```python
from build123d import *

# Parameters (mm, degrees)
SKETCH007_R      = 2.25
EXTRUDE007_DEPTH = 6
SKETCH006_R      = 3
SKETCH006_W      = 15
SKETCH006_H      = 10
EXTRUDE006_DEPTH = 2
SKETCH005_W      = 62
SKETCH005_H      = 5
EXTRUDE005_DEPTH = 2
SKETCH004_W      = 62
SKETCH004_H      = 5
EXTRUDE004_DEPTH = 2
SKETCH003_R      = 1
EXTRUDE003_DEPTH = 4
SKETCH002_R      = 3
EXTRUDE002_DEPTH = 4
SKETCH001_W      = 88
SKETCH001_H      = 84
EXTRUDE001_DEPTH = 29
SKETCH_W         = 91
SKETCH_H         = 87
EXTRUDE_DEPTH    = 29
BOX_W            = 91
BOX_H            = 87
BOX_DEPTH        = 3
FILLET_R         = 2
FILLET001_R      = 2
FILLET002_R      = 2
FILLET003_R      = 2
FILLET004_R      = 2
FILLET005_R      = 2
FILLET006_R      = 2
FILLET007_R      = 2
FILLET008_R      = 2
FILLET009_R      = 2
FILLET010_R      = 2
FILLET011_R      = 2


with BuildPart() as extrude007:
    # Sketch007 (on Face52 of Fillet011) → Extrude007 (new body)
    with BuildSketch(Plane(origin=(0, 0, 0), x_dir=(1, 0, 0), z_dir=(0, 0, -1))):
        with Locations((45.5, -5.25)):
            Circle(SKETCH007_R)
        with Locations((75.5, -5.25)):
            Circle(SKETCH007_R)
        with Locations((15.5, -5.25)):
            Circle(SKETCH007_R)
        with Locations((15.5, -35.25)):
            Circle(SKETCH007_R)
        with Locations((45.5, -35.25)):
            Circle(SKETCH007_R)
        with Locations((75.5, -35.25)):
            Circle(SKETCH007_R)
        with Locations((15.5, -65.25)):
            Circle(SKETCH007_R)
        with Locations((45.5, -65.25)):
            Circle(SKETCH007_R)
        with Locations((75.5, -65.25)):
            Circle(SKETCH007_R)
    extrude(amount=EXTRUDE007_DEPTH)


with BuildPart() as extrude006:
    # Sketch006 (on Face13 of Cut002) → Extrude006 (new body)
    with BuildSketch(Plane(origin=(0, 87, 0), x_dir=(-1, 0, 0), z_dir=(0, 1, 0))):
        with Locations((-64.5, 19.802082)):
            Circle(SKETCH006_R)
        with Locations((-45.5, 22)):
            Rectangle(SKETCH006_W, SKETCH006_H)
    extrude(amount=-EXTRUDE006_DEPTH)


with BuildPart() as extrude005:
    # Sketch005 (on Face17 of Cut001) → Extrude005 (new body)
    with BuildSketch(Plane(origin=(0, 0, 0), x_dir=(0, -1, 0), z_dir=(-1, 0, 0))):
        with Locations((-39, 10.5)):
            Rectangle(SKETCH005_W, SKETCH005_H)
    extrude(amount=-EXTRUDE005_DEPTH)


with BuildPart() as extrude004:
    # Sketch004 (on Face10 of Fusion002) → Extrude004 (new body)
    with BuildSketch(Plane.YZ.offset(91)):
        with Locations((39, 10.5)):
            Rectangle(SKETCH004_W, SKETCH004_H)
    extrude(amount=-EXTRUDE004_DEPTH)


with BuildPart() as extrude003:
    # Sketch003 (on Face34 of Fusion001) → Extrude003 (new body)
    with BuildSketch(Plane.XY.offset(7)):
        with Locations((5.302703, 5.215435)):
            Circle(SKETCH003_R)
        with Locations((85.638989, 5.056605)):
            Circle(SKETCH003_R)
        with Locations((85.765417, 81.797994)):
            Circle(SKETCH003_R)
        with Locations((5.093359, 81.86968)):
            Circle(SKETCH003_R)
    extrude(amount=EXTRUDE003_DEPTH)


with BuildPart() as extrude002:
    # Sketch002 (on Face18 of Fillet007) → Extrude002 (new body)
    with BuildSketch(Plane.XY.offset(3)):
        with Locations((5.093359, 81.86968)):
            Circle(SKETCH002_R)
        with Locations((85.80056, 81.783242)):
            Circle(SKETCH002_R)
        with Locations((5.279273, 5.214621)):
            Circle(SKETCH002_R)
        with Locations((85.631504, 5.092482)):
            Circle(SKETCH002_R)
    extrude(amount=EXTRUDE002_DEPTH)


with BuildPart() as extrude001:
    # Sketch001 (on Face6 of Box) → Extrude001 (new body)
    with BuildSketch(Plane.XY.offset(3)):
        with Locations((45.5, 43.5)):
            Rectangle(SKETCH001_W, SKETCH001_H)
    extrude(amount=EXTRUDE001_DEPTH)


with BuildPart() as cut:
    # Sketch (on Face6 of Box) → Extrude (new body)
    with BuildSketch(Plane.XY.offset(3)):
        with Locations((45.5, 43.5)):
            Rectangle(SKETCH_W, SKETCH_H)
    extrude(amount=EXTRUDE_DEPTH)

    # Cut: cut Extrude001
    add(extrude001.part, mode=Mode.SUBTRACT)


with BuildPart() as esp_case_bottom:
    # Box → Box (new body)
    with BuildSketch(Plane.XY):
        with Locations((45.5, 43.5)):
            Rectangle(BOX_W, BOX_H)
    extrude(amount=BOX_DEPTH)

    # Fusion: union Cut
    add(cut.part)

    # Fillet
    fillet_edges = [esp_case_bottom.edges().sort_by_distance(p)[0] for p in [
        (0, 87, 1.5),
        (0, 87, 17.5),
    ]]
    fillet(fillet_edges, radius=FILLET_R)

    # Fillet001
    fillet001_edges = [esp_case_bottom.edges().sort_by_distance(p)[0] for p in [
        (1.5, 85.5, 17.5),
    ]]
    fillet(fillet001_edges, radius=FILLET001_R)

    # Fillet002
    fillet002_edges = [esp_case_bottom.edges().sort_by_distance(p)[0] for p in [
        (0, 0, 17.5),
    ]]
    fillet(fillet002_edges, radius=FILLET002_R)

    # Fillet003
    fillet003_edges = [esp_case_bottom.edges().sort_by_distance(p)[0] for p in [
        (91, 0, 17.5),
    ]]
    fillet(fillet003_edges, radius=FILLET003_R)

    # Fillet004
    fillet004_edges = [esp_case_bottom.edges().sort_by_distance(p)[0] for p in [
        (91, 87, 17.5),
    ]]
    fillet(fillet004_edges, radius=FILLET004_R)

    # Fillet005
    fillet005_edges = [esp_case_bottom.edges().sort_by_distance(p)[0] for p in [
        (89.5, 85.5, 17.5),
    ]]
    fillet(fillet005_edges, radius=FILLET005_R)

    # Fillet006
    fillet006_edges = [esp_case_bottom.edges().sort_by_distance(p)[0] for p in [
        (89.5, 1.5, 17.5),
    ]]
    fillet(fillet006_edges, radius=FILLET006_R)

    # Fillet007
    fillet007_edges = [esp_case_bottom.edges().sort_by_distance(p)[0] for p in [
        (1.5, 1.5, 17.5),
    ]]
    fillet(fillet007_edges, radius=FILLET007_R)

    # Fusion001: union Extrude002
    add(extrude002.part)

    # Fusion002: union Extrude003
    add(extrude003.part)

    # Cut001: cut Extrude004
    add(extrude004.part, mode=Mode.SUBTRACT)

    # Cut002: cut Extrude005
    add(extrude005.part, mode=Mode.SUBTRACT)

    # Cut003: cut Extrude006
    add(extrude006.part, mode=Mode.SUBTRACT)

    # Fillet008
    fillet008_edges = [esp_case_bottom.edges().sort_by_distance(p)[0] for p in [
        (38, 86.25, 17),
    ]]
    fillet(fillet008_edges, radius=FILLET008_R)

    # Fillet009
    fillet009_edges = [esp_case_bottom.edges().sort_by_distance(p)[0] for p in [
        (53, 86.25, 27),
    ]]
    fillet(fillet009_edges, radius=FILLET009_R)

    # Fillet010
    fillet010_edges = [esp_case_bottom.edges().sort_by_distance(p)[0] for p in [
        (53, 86.25, 17),
    ]]
    fillet(fillet010_edges, radius=FILLET010_R)

    # Fillet011
    fillet011_edges = [esp_case_bottom.edges().sort_by_distance(p)[0] for p in [
        (38, 86.25, 27),
    ]]
    fillet(fillet011_edges, radius=FILLET011_R)

    # Fusion003: union Extrude007
    add(extrude007.part)


solid = esp_case_bottom.part
```
Source: CAD feature listing. Evaluate the final solid. Frame: model axes, mm. A direction names the side the tool comes from. Give positions to 0.01 mm unless a question says otherwise; leave off trailing zeros. Loops run counter-clockwise (first coordinate to the right, second up) from the corner with the lowest first, then second, coordinate; pieces in that order, holes last. Notation, with made-up numbers: (77, -11) -> (90, -11) arc R16 ccw to (90, -3) -> close; hole circle Ø8 at (-1.75, 75.5). An arc over 180 degrees is marked (long way). Put each result on its own line as item: value. Start each with the question number.
1) Cut plane B-B (x = 45.5). Return loops of the section in (y, z).
2) Cut plane A-A (y = 16.5). Return loops of the section in (x, z).
3) Draft query along Y for faces 1 (the face through (1.5, 43, 17)), 2 (the face through (45, 0, 16)), 3 (the face through (45, 5, -6)). Return one class per face: released by +Y, released by -Y, zero draft, split by the parting line, or undercut.
4) Cut plane C-C (z = -3). State how many separate pieces and enclosed holes the cut face has, then the cut area to 3 significant figures.
5) Contact query for flat-ended pins moving along their axis: P1, Ø6.5, axis at x = 86.5, y = 81, coming from the +Z side; P2, Ø1.2, axis at y = 86, z = 23, coming from the +X side; P3, Ø12, axis at x = 55, y = 50.5, coming from the -Z side; P4, Ø1.6, axis at y = 86.5, z = 21, coming from the -X side. Output: stop coordinate, or through.
6) Material intervals for probe 1 along Y at (x, z) = (40, 13.5); probe 2 along X at (y, z) = (23.5, 14); probe 3 along Z at (x, y) = (64.5, 85.8), sorted ascending.
7) Reachability of faces 4 (the face through (52.43, 86.24, 26.4)), 5 (the face through (88.93, 2.1, 17.7)), 6 (the face through (45, 44, 0)) from +Z, -Z, +X, -X, +Y, -Y: full face, straight path, thin tool, end or side. Return the list, or none.
8) Cut plane D-D (z = 14.5). Return loops of the section in (x, y), then the cut area to 3 significant figures.
Results are:
1. outline: (0, 0) -> (3, 0) -> (3, -6) -> (7.5, -6) -> (7.5, 0) -> (33, 0) -> (33, -6) -> (37.5, -6) -> (37.5, 0) -> (63, 0) -> (63, -6) -> (67.5, -6) -> (67.5, 0) -> (87, 0) -> (87, 17) -> (85.5, 17) -> (85.5, 3) -> (1.5, 3) -> (1.5, 32) -> (0, 32) -> close; (85.5, 27) -> (87, 27) -> (87, 32) -> (85.5, 32) -> close
2. outline: (0, 0) -> (91, 0) -> (91, 8) -> (89.5, 8) -> (89.5, 3) -> (1.5, 3) -> (1.5, 8) -> (0, 8) -> close; (0, 13) -> (1.5, 13) -> (1.5, 32) -> (0, 32) -> close; (89.5, 13) -> (91, 13) -> (91, 32) -> (89.5, 32) -> close
3. face 1: undercut
3. face 2: released by -Y
3. face 3: zero draft
4. separate pieces: 9
4. enclosed holes: 0
4. area: 143 mm2
5. P1: stops at z = 32
5. P2: stops at x = 90.96
5. P3: stops at z = 0
5. P4: stops at x = 0.13
6. probe 1: y = 0 to 1.5, 85.5 to 87
6. probe 2: x = 0 to 1.5, 89.5 to 91
6. probe 3: z = 0 to 16.8, 22.8 to 32
7. face 4: +Y
7. face 5: +Z
7. face 6: -Z
8. outline: (0, 2) arc R2 ccw to (2, 0) -> (89, 0) arc R2 ccw to (91, 2) -> (91, 85) arc R2 ccw to (89, 87) -> (2, 87) arc R2 ccw to (0, 85) -> close; hole (1.5, 3.5) arc R2 ccw to (3.5, 1.5) -> (87.5, 1.5) arc R2 ccw to (89.5, 3.5) -> (89.5, 83.5) arc R2 ccw to (87.5, 85.5) -> (3.5, 85.5) arc R2 ccw to (1.5, 83.5) -> close
8. area: 525 mm2
